Input: part model. Units: mm. Frame: model coordinates. Coordinates: 2 decimals unless noted, no trailing zeros. Write each loop counter-clockwise with the first axis right and the second up, starting at its lowest first coordinate (ties: lowest second). Pieces come first, ordered by that corner, then holes. Notation, with made-up numbers: M 59.25,-34.5 L 82.25,-34.5 A30 cw 82.25,-0.5 Z; hole C 84.25,79 d1. An arc over 180 degrees is marked long. Use CSV: the item, a comma, the result in double quotes.
```python
from build123d import *

# Parameters (mm, degrees)
F0_W     = 19.05
F0_H     = 152.4
F0_W_2   = 304.8
F0_H_2   = 38.1
F1_DEPTH = 19.05


# Not quite as in the source:
# - a feature names something its author has since deleted; it is built from what else it names


with BuildPart() as f1:
    # F0 (on Front) → F1 (new body)
    with BuildSketch(Plane.XZ):
        Polygon((-438.15, -314.325), (-438.15, -447.675), (-152.4, -447.675), (152.4, -447.675), (438.15, -447.675), (438.15, -314.325), (438.15, -161.925), (438.15, 142.875), (438.15, 295.275), (438.15, 447.675), (357.7166666667, 447.675), (357.7166666667, 422.275), (338.6666666667, 422.275), (338.6666666667, 447.675), (258.2333333333, 447.675), (258.2333333333, 422.275), (239.1833333333, 422.275), (239.1833333333, 447.675), (158.75, 447.675), (158.75, 422.275), (139.7, 422.275), (139.7, 447.675), (59.266836, 447.675), (59.266836, 422.275), (40.216836, 422.275), (40.216836, 447.675), (-40.216836, 447.675), (-40.216836, 422.275), (-59.266836, 422.275), (-59.266836, 447.675), (-139.7, 447.675), (-139.7, 422.275), (-158.75, 422.275), (-158.75, 447.675), (-239.1833333333, 447.675), (-239.1833333333, 422.275), (-258.2333333333, 422.275), (-258.2333333333, 447.675), (-338.6666666667, 447.675), (-338.6666666667, 422.275), (-357.7166666667, 422.275), (-357.7166666667, 447.675), (-438.15, 447.675), (-438.15, 295.275), (-438.15, 142.875), (-438.15, -161.925), align=None)
        Polygon((-304.8, -47.625), (-304.8, -34.925), (-304.8, 41.275), (304.8, 41.275), (304.8, -34.925), (304.8, -47.625), (285.75, -47.625), (285.75, -34.925), (206.375, -34.925), (206.375, -47.625), (187.325, -47.625), (187.325, -34.925), (107.95, -34.925), (107.95, -47.625), (88.9, -47.625), (88.9, -34.925), (9.525, -34.925), (9.525, -47.625), (-9.525, -47.625), (-9.525, -34.925), (-88.9, -34.925), (-88.9, -47.625), (-107.95, -47.625), (-107.95, -34.925), (-187.325, -34.925), (-187.325, -47.625), (-206.375, -47.625), (-206.375, -34.925), (-285.75, -34.925), (-285.75, -47.625), align=None, mode=Mode.SUBTRACT)
        Polygon((-304.8, 295.275), (304.8, 295.275), (304.8, 219.075), (304.8, 206.375), (285.75, 206.375), (285.75, 219.075), (206.375, 219.075), (206.375, 206.375), (187.325, 206.375), (187.325, 219.075), (107.95, 219.075), (107.95, 206.375), (88.9, 206.375), (88.9, 219.075), (9.525, 219.075), (9.525, 206.375), (-9.525, 206.375), (-9.525, 219.075), (-88.9, 219.075), (-88.9, 206.375), (-107.95, 206.375), (-107.95, 219.075), (-187.325, 219.075), (-187.325, 206.375), (-206.375, 206.375), (-206.375, 219.075), (-285.75, 219.075), (-285.75, 206.375), (-304.8, 206.375), (-304.8, 219.075), align=None, mode=Mode.SUBTRACT)
        with Locations((-447.675, 219.075)):
            Rectangle(F0_W, F0_H)
        with Locations((-447.675, -238.125)):
            Rectangle(F0_W, F0_H)
        with Locations((447.675, 219.075)):
            Rectangle(F0_W, F0_H)
        with Locations((447.675, -238.125)):
            Rectangle(F0_W, F0_H)
        with Locations((0, -466.725)):
            Rectangle(F0_W_2, F0_H_2)
    extrude(amount=F1_DEPTH)


solid = f1.part
```
1. Section A-A (x = 274). Return loops of the section in (y, z) (3 decimals).
Resolved:
outline,"M -19.05,-447.675 L 0,-447.675 L 0,-34.925 L -19.05,-34.925 Z; M -19.05,41.275 L 0,41.275 L 0,219.075 L -19.05,219.075 Z; M -19.05,295.275 L 0,295.275 L 0,447.675 L -19.05,447.675 Z"
2. Section D-D (z = 281). Return loops of the section in (x, y).
Resolved:
outline,"M -457.2,-19.05 L -304.8,-19.05 L -304.8,0 L -457.2,0 Z; M 304.8,-19.05 L 457.2,-19.05 L 457.2,0 L 304.8,0 Z"
3. Section B-B (z = 1). Return loops of the section in (x, y).
Resolved:
outline,"M -438.15,-19.05 L -304.8,-19.05 L -304.8,0 L -438.15,0 Z; M 304.8,-19.05 L 438.15,-19.05 L 438.15,0 L 304.8,0 Z"
4. Contact query for flat-ended pins moving along their axis: pin 1 Ø9.5 at (x, y) = (-148.5, -9) entering from +Z (3 decimals); pin 2 Ø5 at (y, z) = (-7, -33.5) entering from -X; pin 3 Ø10 at (x, y) = (352.5, -12.5) entering from -Z (3 decimals). Output: stop coordinate, or through.
Resolved:
pin 1,"stops at z = 422.275"
pin 2,"stops at x = -438.15"
pin 3,"stops at z = -447.675"
5. Section C-C (y = -6.5). State how many separate pieces and enclosed holes the cut face has, then the cut area to 3 significant figures.
Resolved:
separate pieces,"1"
enclosed holes,"2"
area,"708,000 mm^2"
6. Material intervals for line 1 (Z direction, x = 23, y = -13.25) (3 decimals); line 2 (Z direction, x = -262.5, y = -2.25) (3 decimals); line 3 (X direction, y = -16, z = -19), sorted ascending. Write a range as [from, to].
Resolved:
line 1,"z = [-485.775, -34.925], [41.275, 219.075], [295.275, 447.675]"
line 2,"z = [-447.675, -34.925], [41.275, 219.075], [295.275, 447.675]"
line 3,"x = [-438.15, -304.8], [304.8, 438.15]"
